Source: CAD feature listing. Evaluate the final solid. Frame: model axes, mm. Round coordinates to 2 decimals unless told otherwise and drop trailing zeros. Order: outer loops, then holes, each group sorted by start corner. A loop starts at its lowest first (then second) coordinate and runs counter-clockwise, first axis right, second up. Notation, with made-up numbers: (-40, 89.25) -> (-26, 89.25) arc R30 cw to (-26, 125.25) -> close; hole circle Ø9 at (-32, 52). An arc over 180 degrees is marked (long way). One line per item, written item: value. Start each with the question number.
1) Ray query, L1, parallel to Z at x = -8, y = 7.05; L2, parallel to Y at x = 6, z = 9.5; L3, parallel to Z at x = -5, y = 270.2. Return the intervals inside material, ascending.
2) Section A-A (y = 270.2). Return the cut outline in (x, z).
3) Pin query (flat end, axial travel): P1, Ø6, axis at x = 1, z = 10, coming from the -Y side; P2, Ø3, axis at y = 7.05, z = 5, coming from the -X side. Return the tip coordinate at first contact, or that it passes through.
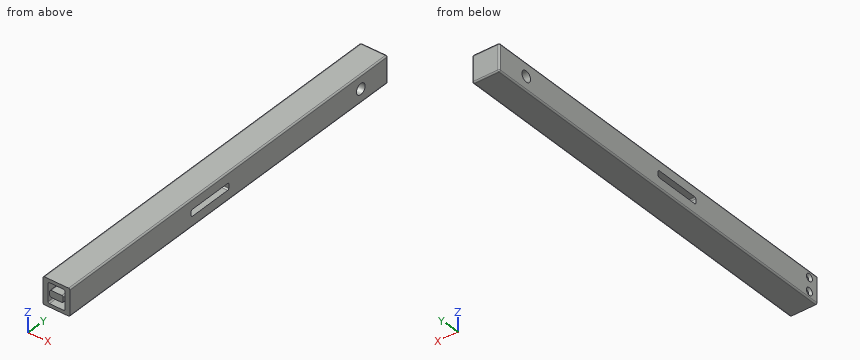
```python
from build123d import *

# Parameters (mm, degrees)
SKETCH1_W                       = 20
SKETCH1_H                       = 295.2
BOSS_EXTRUDE1_DEPTH             = 20
CUT_EXTRUDE1_REACH              = 298.552
SKETCH2_R                       = 4
CUT_EXTRUDE2_DEPTH              = 14.1
CUT_EXTRUDE3_DEPTH              = 297.551917883
M3X0_5_TAPPED_HOLE1_D           = 2.5
M3X0_5_TAPPED_HOLE1_DEPTH       = 18
M3X0_5_TAPPED_HOLE1_CSINK_D     = 5.6
M3X0_5_TAPPED_HOLE1_CSINK_ANGLE = 90
M3X0_5_TAPPED_HOLE1_TIP         = 0.751075774
FILLET1_R                       = 1
FILLET2_R                       = 1


with BuildPart() as part:
    # Sketch1 → Boss-Extrude1 (new body)
    with BuildSketch(Plane.XY):
        with Locations((0, 147.6)):
            Rectangle(SKETCH1_W, SKETCH1_H)
    extrude(amount=BOSS_EXTRUDE1_DEPTH)

    # Sketch2 → Cut-Extrude1 (cut, up to next)
    with BuildSketch(Plane(origin=(10, 0, 0), x_dir=(0, 0, -1), z_dir=(1, 0, 0)), mode=Mode.PRIVATE) as cut_extrude1_sk1:
        with Locations(Location((-10, 270.2, 0), (0, 0, 90))):
            Circle(SKETCH2_R)
    cut_extrude1_tool1 = extrude(cut_extrude1_sk1.sketch, amount=-CUT_EXTRUDE1_REACH, mode=Mode.PRIVATE) & part.part
    add(cut_extrude1_tool1.solids().sort_by_distance((10, 270.2, 10))[0], mode=Mode.SUBTRACT)

    # Sketch3 → Cut-Extrude2 (cut)
    with BuildSketch(Plane.XZ):
        with BuildLine():
            Line((-5.25, 2.5), (5.25, 2.5))
            ThreePointArc((5.25, 2.5), (5.957106781, 2.792893219), (6.25, 3.5))
            Line((6.25, 3.5), (6.25, 16.5))
            ThreePointArc((6.25, 16.5), (5.957106781, 17.207106781), (5.25, 17.5))
            Line((5.25, 17.5), (-5.25, 17.5))
            ThreePointArc((-5.25, 17.5), (-5.957106781, 17.207106781), (-6.25, 16.5))
            Line((-6.25, 16.5), (-6.25, 3.5))
            ThreePointArc((-6.25, 3.5), (-5.957106781, 2.792893219), (-5.25, 2.5))
        make_face()
        with BuildLine():
            Line((-4, 7.5), (4, 7.5))
            ThreePointArc((4, 7.5), (4.707106781, 7.792893219), (5, 8.5))
            Line((5, 8.5), (5, 11.5))
            ThreePointArc((5, 11.5), (4.707106781, 12.207106781), (4, 12.5))
            Line((4, 12.5), (-4, 12.5))
            ThreePointArc((-4, 12.5), (-4.707106781, 12.207106781), (-5, 11.5))
            Line((-5, 11.5), (-5, 8.5))
            ThreePointArc((-5, 8.5), (-4.707106781, 7.792893219), (-4, 7.5))
        make_face(mode=Mode.SUBTRACT)
    extrude(amount=-CUT_EXTRUDE2_DEPTH, mode=Mode.SUBTRACT)

    # Sketch5 → Cut-Extrude3 (cut, through all)
    with BuildSketch(Plane.ZY.offset(10)):
        with BuildLine():
            Line((8.5, 147.6), (11.5, 147.6))
            ThreePointArc((11.5, 147.6), (12.207106781, 147.307106781), (12.5, 146.6))
            Line((12.5, 146.6), (12.5, 113.6))
            ThreePointArc((12.5, 113.6), (12.207106781, 112.892893219), (11.5, 112.6))
            Line((11.5, 112.6), (8.5, 112.6))
            ThreePointArc((8.5, 112.6), (7.792893219, 112.892893219), (7.5, 113.6))
            Line((7.5, 113.6), (7.5, 146.6))
            ThreePointArc((7.5, 146.6), (7.792893219, 147.307106781), (8.5, 147.6))
        make_face()
    extrude(amount=-CUT_EXTRUDE3_DEPTH, mode=Mode.SUBTRACT)

    # M3x0.5 Tapped Hole1
    with Locations(Plane.ZY.offset(10)):
        with Locations((15, 7.05), (5, 7.05)):
            CounterSinkHole(M3X0_5_TAPPED_HOLE1_D / 2, M3X0_5_TAPPED_HOLE1_CSINK_D / 2, depth=M3X0_5_TAPPED_HOLE1_DEPTH, counter_sink_angle=M3X0_5_TAPPED_HOLE1_CSINK_ANGLE)
            with Locations((0, 0, -(M3X0_5_TAPPED_HOLE1_DEPTH + M3X0_5_TAPPED_HOLE1_TIP / 2))):  # 118° drill point
                Cone(0, M3X0_5_TAPPED_HOLE1_D / 2, M3X0_5_TAPPED_HOLE1_TIP, mode=Mode.SUBTRACT)

    # Fillet1
    fillet1_edges = [part.edges().sort_by_distance(p)[0] for p in [
        (-10, 295.2, 10),
        (10, 295.2, 10),
    ]]
    fillet(fillet1_edges, radius=FILLET1_R)

    # Fillet2
    fillet2_edges = [part.edges().sort_by_distance(p)[0] for p in [
        (10, 147.1, 20),
        (0, 295.2, 0),
        (0, 295.2, 20),
        (-10, 147.1, 0),
        (-9.707106781, 294.907106781, 0),
        (9.707106781, 294.907106781, 0),
        (-10, 147.1, 20),
        (-9.707106781, 294.907106781, 20),
        (9.707106781, 294.907106781, 20),
        (10, 147.1, 0),
    ]]
    fillet(fillet2_edges, radius=FILLET2_R)


solid = part.part
```
Findings:
1. L1: 0 to 3.75, 6.25 to 13.75, 16.25 to 20
1. L2: 14.1 to 112.6, 147.6 to 266.23, 274.17 to 295.2
1. L3: 0 to 6, 14 to 20
2. outline: (-10, 1) arc R1 ccw to (-9, 0) -> (9, 0) arc R1 ccw to (10, 1) -> (10, 6) -> (-10, 6) -> close; (-10, 14) -> (10, 14) -> (10, 19) arc R1 ccw to (9, 20) -> (-9, 20) arc R1 ccw to (-10, 19) -> close
3. P1: y = 0
3. P2: x = -8.7
